Part print with two shaded views. Sizes in mm from the minimum x, y, z corner. A direction names the side the tool comes from. Coordinates: 2 decimals unless noted, no trailing zeros. Loops run counter-clockwise (first coordinate to the right, second up) from the corner with the lowest first, then second, coordinate; pieces in that order, holes last.
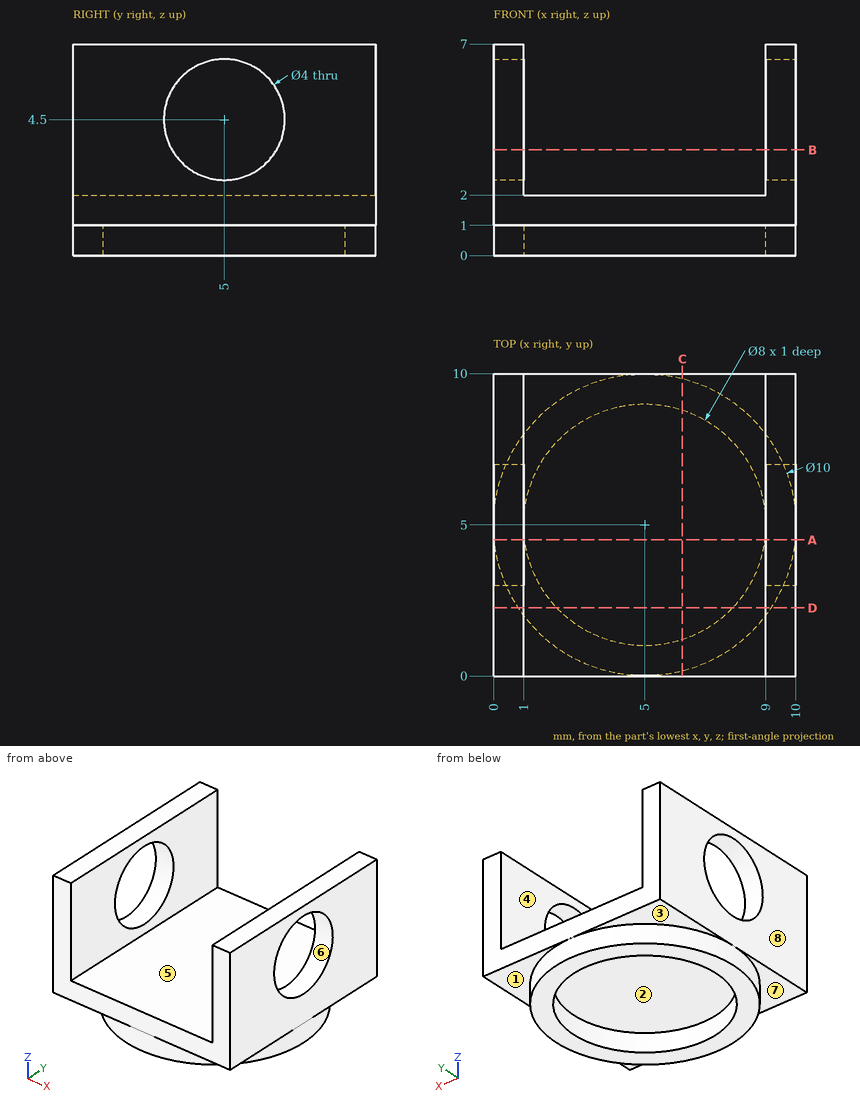
Q1. Slice it at C-C (x = 6.25). List the corners of the cut face in (y, z).
Answers:
outline: (0, 1) - (0.16, 1) - (0.16, 0) - (1.2, 0) - (1.2, 1) - (8.8, 1) - (8.8, 0) - (9.84, 0) - (9.84, 1) - (10, 1) - (10, 2) - (0, 2) - close
Q2. Flat gauge pins, fed straight in: P1, Ø3, axis at y = 5, z = 4.5, coming from the -X side; P2, Ø2.5, axis at x = 4, y = 4, coming from the +Z side; P3, Ø2.5, axis at x = 3.5, y = 5, coming from the -Z side. Where does each tip first touch, or does it go through?
Answers:
P1: passes through
P2: stops at z = 2
P3: stops at z = 1
Q3. Which spindle directions (+Z, -Z, +X, -X, +Y, -Y) get a long thin tool onto all of the face, cutting with end or side? Do the marked faces 1, 2, 3 and 4. Say none if no direction does.
Answers:
face 1: -Z, +X, +Y
face 2: -Z
face 3: -Z, -X, +Y
face 4: +Z, +Y, -Y
Q4. Slice it at B-B (z = 3.5). List the corners of the cut face in (x, y).
Answers:
outline: (0, 0) - (1, 0) - (1, 3.27) - (0, 3.27) - close; (0, 6.73) - (1, 6.73) - (1, 10) - (0, 10) - close; (9, 0) - (10, 0) - (10, 3.27) - (9, 3.27) - close; (9, 6.73) - (10, 6.73) - (10, 10) - (9, 10) - close
Q5. Slice it at D-D (y = 2.25). List the corners of the cut face in (x, z), and give its area (3 significant figures).
Answers:
outline: (0, 1) - (0.82, 1) - (0.82, 0) - (2.1, 0) - (2.1, 1) - (7.9, 1) - (7.9, 0) - (9.18, 0) - (9.18, 1) - (10, 1) - (10, 7) - (9, 7) - (9, 2) - (1, 2) - (1, 7) - (0, 7) - close
area: 22.5 mm2
Q6. Slice it at A-A (y = 4.5). Count the separate pieces of the cut face and the enclosed holes in it, and give its area (3 significant figures).
Answers:
separate pieces: 3
enclosed holes: 0
area: 14.3 mm2
Q7. Drill centre lines: line 1 (Y direction, x = 5, z = 0.25); line 2 (Y direction, x = 0.65, z = 4.5). Where is each one in solid material? Low to high.
Answers:
line 1: y = 0 to 1, 9 to 10
line 2: y = 0 to 3, 7 to 10
Q8. Mould opens along Z. For the marked faces 5, 6, 7 and 8 say: +Z half, -Z half, draft (parallel to the pull), parting line (faces both ways), or undercut.
Answers:
face 5: +Z half
face 6: undercut
face 7: -Z half
face 8: draft
